from build123d import *

# Parameters (mm, degrees)
F0_R     = 2.6
F1_DEPTH = 7
F2_R     = 3


# Not quite as in the source:
# - a feature names something its author has since deleted; it is built from what else it names


with BuildPart() as f1:
    # F0 (on Front) → F1 (new body)
    with BuildSketch(Plane.XZ):
        with BuildLine():
            ThreePointArc((-19.5484192549, -21.4210014853), (11.706746807, -26.5320952659), (29, 0))
            ThreePointArc((29, 0), (11.706746807, 26.5320952659), (-19.5484192549, 21.4210014853))
            ThreePointArc((-19.5484192549, 21.4210014853), (-24.7548164348, 15.1062590762), (-27.9895839317, 7.5883589353))
            ThreePointArc((-27.9895839317, 7.5883589353), (-29, 0), (-27.9895839317, -7.5883589353))
            ThreePointArc((-27.9895839317, -7.5883589353), (-24.7548164348, -15.1062590762), (-19.5484192549, -21.4210014853))
        make_face()
        Circle(F0_R, mode=Mode.SUBTRACT)
        with BuildLine():
            ThreePointArc((-27.9895839317, 7.5883589353), (-24.7548164348, 15.1062590762), (-19.5484192549, 21.4210014853))
            ThreePointArc((-19.5484192549, 21.4210014853), (-26.7826801614, 20.9280500488), (-33.9694734381, 21.8911359117))
            ThreePointArc((-33.9694734381, 21.8911359117), (-38.616718272, 19.4692528721), (-36.8782865714, 14.5255440189))
            ThreePointArc((-36.8782865714, 14.5255440189), (-32.1832277785, 11.3781861206), (-27.9895839317, 7.5883589353))
        make_face()
        with BuildLine():
            ThreePointArc((-34.8963290453, 16.45), (-36.4463290453, 18), (-34.8963290453, 19.55))
            Line((-34.8963290453, 19.55), (-30.8963290453, 19.55))
            ThreePointArc((-30.8963290453, 19.55), (-29.3463290453, 18), (-30.8963290453, 16.45))
            Line((-30.8963290453, 16.45), (-34.8963290453, 16.45))
        make_face(mode=Mode.SUBTRACT)
        with BuildLine():
            ThreePointArc((-33.9694734381, -21.8911359117), (-26.7826801614, -20.9280500488), (-19.5484192549, -21.4210014853))
            ThreePointArc((-19.5484192549, -21.4210014853), (-24.7548164348, -15.1062590762), (-27.9895839317, -7.5883589353))
            ThreePointArc((-27.9895839317, -7.5883589353), (-32.1832277785, -11.3781861206), (-36.8782865714, -14.5255440189))
            ThreePointArc((-36.8782865714, -14.5255440189), (-38.616718272, -19.4692528721), (-33.9694734381, -21.8911359117))
        make_face()
        with BuildLine():
            Line((-34.8963290453, -16.45), (-30.8963290453, -16.45))
            ThreePointArc((-30.8963290453, -16.45), (-29.3463290453, -18), (-30.8963290453, -19.55))
            Line((-30.8963290453, -19.55), (-34.8963290453, -19.55))
            ThreePointArc((-34.8963290453, -19.55), (-36.4463290453, -18), (-34.8963290453, -16.45))
        make_face(mode=Mode.SUBTRACT)
    extrude(amount=F1_DEPTH)

    # F2 (on Right) → F3 (revolve, cut)
    with BuildSketch(Plane.YZ):
        with Locations((-7.5, 25)):
            Circle(F2_R)
    revolve(axis=Axis((0, 0, 0), (0, -1, 0)), mode=Mode.SUBTRACT)


solid = f1.part
Input: part model. Units: mm. Frame: model coordinates. A direction names the side the tool comes from. Give positions to 0.01 mm unless a question says otherwise; leave off trailing zeros. Write each loop counter-clockwise with the first axis right and the second up, starting at its lowest first coordinate (ties: lowest second). Pieces come first, ordered by that corner, then holes. Notation, with made-up numbers: M 68,-0.75 L 89,-0.75 A21 cw 89,17.25 Z; hole C 3.25,-5.75 d11. An arc over 180 degrees is marked long. Write item = value, one per line. Start each with the question number.
1) Cut plane C-C on y = -2. Return the cut outline in (x, z).
2) Draft query along X for faces 4 (the cylindrical face through (-32.12, -3.45, -11.33)), 5 (the flat face through (-33, -3, -19.55)), 6 (the cylindrical face through (-26.88, -3.45, -20.93)), 7 (the flat face through (0, -7, -5)). Return one class per face: +X half, -X half, draft (parallel to the pull), parting line (faces both ways), or undercut.
3) Material intervals for line 1 along Z through (x, y) = (0, -2.5); line 2 along X through (y, z) = (-5.5, 17); line 3 along Z through (x, y) = (0, -4.75), sorted ascending. Write a range as [from, to].
4) First-contact query: pin 1 Ø4.5 at (x, z) = (0, 0) entering from -Y; pin 2 Ø3 at (x, y) = (-33.5, -4.5) entering from +Z; pin 3 Ø4 at (x, y) = (-6, -5) entering from -Z; pin 4 Ø1 at (x, y) = (-9.5, -1.5) entering from +Z. Flat tips, straight axial feed; report the tip coordinate or a pass-through.
5) Cut plane A-A on x = 0. Return the cut outline in (y, z), then the cut area to 3 significant figures.
6) Reachability of faces 1 (the flat face through (-28, -7, 4)), 2 (the cylindrical face through (-32.25, -3.45, 11.43)), 3 (the flat face through (-33, -3, 19.55)) from +Z, -Z, +X, -X, +Y, -Y: full face, straight path, thin tool, end or side. Return the list, or none.
7) Cut plane B-B on y = -6. Return the cut outline in (x, z).
Solved:
q1.outline = M -36.88,-14.53 A4 ccw -33.97,-21.89 A36.09 cw -19.55,-21.42 A29 ccw long -19.55,21.42 A36.09 cw -33.97,21.89 A4 ccw -36.88,14.53 A39.2 cw -27.99,7.59 A29 ccw -27.99,-7.59 A39.2 cw Z; hole M -34.9,-19.55 L -30.9,-19.55 A1.55 ccw -30.9,-16.45 L -34.9,-16.45 A1.55 ccw Z; hole M -34.9,16.45 L -30.9,16.45 A1.55 ccw -30.9,19.55 L -34.9,19.55 A1.55 ccw Z; hole C 0,0 d5.2
q2.face_4 = -X half
q2.face_5 = undercut
q2.face_6 = undercut
q2.face_7 = draft
q3.line_1 = [-29, -2.6], [2.6, 29]
q3.line_2 = [-38.77, -36.08], [-29.71, -21.28], [-15.14, 15.14], [21.28, 23.49]
q3.line_3 = [-29, -26.2], [-23.8, -2.6], [2.6, 23.8], [26.2, 29]
q4.pin_1 = through
q4.pin_2 = 22
q4.pin_3 = -28.72
q4.pin_4 = 27.57
q5.outline = M -7,-29 L 0,-29 L 0,-2.6 L -7,-2.6 L -7,-22.04 A3 cw -7,-27.96 Z; M -7,2.6 L 0,2.6 L 0,29 L -7,29 L -7,27.96 A3 cw -7,22.04 Z
q5.area = 347 mm2
q6.face_1 = +Z, -Z, +X, -X, -Y
q6.face_2 = -X, +Y, -Y
q6.face_3 = +Y, -Y
q7.outline = M -36.88,-14.53 A4 ccw -33.97,-21.89 A36.09 cw -19.55,-21.42 A29 ccw long -19.55,21.42 A36.09 cw -33.97,21.89 A4 ccw -36.88,14.53 A39.2 cw -27.99,7.59 A29 ccw -27.99,-7.59 A39.2 cw Z; C 0,0 d44.8; hole M -34.9,-19.55 L -30.9,-19.55 A1.55 ccw -30.9,-16.45 L -34.9,-16.45 A1.55 ccw Z; hole M -34.9,16.45 L -30.9,16.45 A1.55 ccw -30.9,19.55 L -34.9,19.55 A1.55 ccw Z; hole C 0,0 d55.2; hole C 0,0 d5.2
